```python
from build123d import *

# Parameters (mm, degrees)
F0_W     = 177.8
F0_H     = 177.8
F1_DEPTH = 177.8
F2_W     = 174.625
F2_H     = 171.45
F3_DEPTH = 174.625
F4_R     = 40.471876


with BuildPart() as f1:
    # F0 (on Top) → F1 (new body)
    with BuildSketch(Plane.XY):
        Rectangle(F0_W, F0_H)
    extrude(amount=F1_DEPTH)

    # F2 (on face) → F3 (cut)
    with BuildSketch(Plane.XY.offset(177.8)):
        with Locations((1.5875, 0)):
            Rectangle(F2_W, F2_H)
    extrude(amount=-F3_DEPTH, mode=Mode.SUBTRACT)

    # F4
    f4_edges = [f1.edges().sort_by_distance(p)[0] for p in [
        (1.5875, 85.725, 3.175),
        (-85.725, 85.725, 90.4875),
        (-85.725, 0, 3.175),
        (-85.725, -85.725, 90.4875),
        (1.5875, -85.725, 3.175),
    ]]
    fillet(f4_edges, radius=F4_R)


solid = f1.part
```
Can you work these out from the model? Positions are in its coordinate system, mm. A direction names the side the tool comes from. Round coordinates to 2 decimals unless told otherwise and drop trailing zeros. Loops run counter-clockwise (first coordinate to the right, second up) from the corner with the lowest first, then second, coordinate; pieces in that order, holes last. Notation, with made-up numbers: (68.5, 74.25) -> (88.5, 74.25) arc R23 ccw to (88.5, 93.25) -> close; hole circle Ø1 at (54, -36.75). An arc over 180 degrees is marked (long way). Answer in a Markdown table with one row per item.
Item 1: Suppose I cut it at B-B, the plane x = -21. List the corners of the cut face in (y, z) for me (3 decimals).
Answer block:
| item | result |
|---|---|
| outline | (-88.9, 0) -> (88.9, 0) -> (88.9, 177.8) -> (85.725, 177.8) -> (85.725, 43.647) arc R40.472 cw to (45.253, 3.175) -> (-45.253, 3.175) arc R40.472 cw to (-85.725, 43.647) -> (-85.725, 177.8) -> (-88.9, 177.8) -> close |
Item 2: On a 3-axis mill with a long thin cutter (end or side, diameter ignored), from which of +Z, -Z, +X, -X, +Y, -Y can I reach the whole of each face in a straight line? I mean faces 4 (the flat face through (21, 1, 3.175)), 5 (the flat face through (-88.9, -1, 88)). Say none if no direction works.
Answer block:
| item | result |
|---|---|
| face 4 | +Z, +X |
| face 5 | +Z, -Z, -X, +Y, -Y |
Item 3: Will these pins go through, and if not, where does the flat tip stop? P1, Ø2, axis at x = 25, y = -63, coming from the +Z side; P2, Ø5, axis at x = 20, y = -13, coming from the -Z side; P3, Ø2, axis at y = 47, z = 62, coming from the +X side; P4, Ø12, axis at x = 30.5, y = -0.5, coming from the +Z side (3 decimals).
Answer block:
| item | result |
|---|---|
| P1 | z = 7.78 |
| P2 | z = 0 |
| P3 | x = -85.63 |
| P4 | z = 3.175 |
Item 4: Suppose I cut it at C-C, the plane z = 157. List the corners of the cut face in (x, y) for me (3 decimals), plus the area to 3 significant figures.
Answer block:
| item | result |
|---|---|
| outline | (-88.9, -88.9) -> (88.9, -88.9) -> (88.9, -85.725) -> (-45.253, -85.725) arc R40.472 cw to (-85.725, -45.253) -> (-85.725, 45.253) arc R40.472 cw to (-45.253, 85.725) -> (88.9, 85.725) -> (88.9, 88.9) -> (-88.9, 88.9) -> close |
| area | 2,380 mm² |
Item 5: Suppose I cut it at A-A, the plane y = 12. List the corners of the cut face in (x, z) for me (3 decimals).
Answer block:
| item | result |
|---|---|
| outline | (-88.9, 0) -> (88.9, 0) -> (88.9, 3.175) -> (-45.253, 3.175) arc R40.472 cw to (-85.725, 43.647) -> (-85.725, 177.8) -> (-88.9, 177.8) -> close |
Item 6: If I drill on probe 1 along Y at (x, z) = (-16, 103) (3 decimals); probe 2 along X at (y, z) = (13, 145) (3 decimals); probe 3 along Z at (x, y) = (44, 13) (3 decimals), over which ranges is the centre line in solid material (lowest first)?
Answer block:
| item | result |
|---|---|
| probe 1 | -88.9 to -85.725, 85.725 to 88.9 |
| probe 2 | -88.9 to -85.725 |
| probe 3 | 0 to 3.175 |
Item 7: We'd pull the mould along Z, two halves only. Please class faces 1 (the flat face through (-1, 1, 0)), 2 (the cylindrical face through (22.763, 74.184, 15.345)), 3 (the flat face through (-1, -88.9, 88)): released by +Z, released by -Z, zero draft, split by the parting line, or undercut.
Answer block:
| item | result |
|---|---|
| face 1 | released by -Z |
| face 2 | released by +Z |
| face 3 | zero draft |
Item 8: Suppose I cut it at D-D, the plane y = -56. List the corners of the cut face in (x, z) for me.
Answer block:
| item | result |
|---|---|
| outline | (-88.9, 0) -> (88.9, 0) -> (88.9, 4.63) -> (-45.25, 4.63) arc R39.02 cw to (-84.27, 43.65) -> (-84.27, 177.8) -> (-88.9, 177.8) -> close |
